```python
from build123d import *

# Parameters (mm, degrees)
RESSALTO_EXTRUS_O1_DEPTH = 8
ESBO_O2_W                = 2.8
ESBO_O2_H                = 2.8
CORTE_EXTRUS_O2_DEPTH    = 20.45530599


with BuildPart() as part:
    # Esboço1 → Ressalto-extrusão1 (new body)
    with BuildSketch(Plane.XY):
        with BuildLine():
            Line((0, 0), (-4.7, 0))
            Line((-4.7, 0), (-4.7, -2.5))
            Line((-4.7, -2.5), (-0.2, -2.5))
            Line((-0.2, -2.5), (14.8, -2.5))
            Line((14.8, -2.5), (14.8, 0))
            Line((14.8, 0), (13.3, 0))
            Line((13.3, 0), (13.3, 6))
            ThreePointArc((13.3, 6), (13, 7.270820393), (12.7, 6))
            Line((12.7, 6), (12.7, 0))
            Line((12.7, 0), (11.4, 0))
            Line((11.4, 0), (11.4, 6))
            ThreePointArc((11.4, 6), (11.1, 7.270820393), (10.8, 6))
            Line((10.8, 6), (10.8, 0))
            Line((10.8, 0), (9.5, 0))
            Line((9.5, 0), (9.5, 6))
            ThreePointArc((9.5, 6), (9.2, 7.270820393), (8.9, 6))
            Line((8.9, 6), (8.9, 0))
            Line((8.9, 0), (7.6, 0))
            Line((7.6, 0), (7.6, 6))
            ThreePointArc((7.6, 6), (7.3, 7.270820393), (7, 6))
            Line((7, 6), (7, 0))
            Line((7, 0), (5.7, 0))
            Line((5.7, 0), (5.7, 6))
            ThreePointArc((5.7, 6), (5.4, 7.270820393), (5.1, 6))
            Line((5.1, 6), (5.1, 0))
            Line((5.1, 0), (3.8, 0))
            Line((3.8, 0), (3.8, 6))
            ThreePointArc((3.8, 6), (3.5, 7.270820393), (3.2, 6))
            Line((3.2, 6), (3.2, 0))
            Line((3.2, 0), (1.9, 0))
            Line((1.9, 0), (1.3, 0))
            Line((1.3, 0), (0, 0))
        make_face()
    extrude(amount=RESSALTO_EXTRUS_O1_DEPTH)

    # Esboço2 → Corte-extrusão2 (cut, through all)
    with BuildSketch(Plane.XZ.offset(2.5)):
        with BuildLine():
            Line((-2.7, 8), (-4.7, 8))
            Line((-4.7, 8), (-4.7, 6))
            ThreePointArc((-4.7, 6), (-4.114213562, 7.414213562), (-2.7, 8))
        make_face()
        with BuildLine():
            Line((-4.7, 2), (-4.7, 0))
            Line((-4.7, 0), (-2.7, 0))
            ThreePointArc((-2.7, 0), (-4.114213562, 0.585786438), (-4.7, 2))
        make_face()
        with Locations((-0.7, 4)):
            Rectangle(ESBO_O2_W, ESBO_O2_H)
        with BuildLine():
            Line((13.8, 8), (14.8, 8))
            Line((14.8, 8), (14.8, 7))
            ThreePointArc((14.8, 7), (14.507106781, 7.707106781), (13.8, 8))
        make_face()
        with BuildLine():
            Line((13.8, 0), (14.8, 0))
            Line((14.8, 0), (14.8, 1))
            ThreePointArc((14.8, 1), (14.507106781, 0.292893219), (13.8, 0))
        make_face()
    extrude(amount=-CORTE_EXTRUS_O2_DEPTH, mode=Mode.SUBTRACT)


solid = part.part
```
For this review, take the finished solid that the model builds, in its own axes (mm). A direction names the side the tool comes from. Give positions to 0.01 mm unless a question says otherwise; leave off trailing zeros. Write each loop counter-clockwise with the first axis right and the second up, starting at its lowest first coordinate (ties: lowest second). Pieces come first, ordered by that corner, then holes.
Item 1: Wall thickness on probe 1 along X at (y, z) = (0.75, 1.75); probe 2 along X at (y, z) = (-1, 5.25); probe 3 along Z at (x, y) = (-2, -2): over which ranges is each line inside the solid? List them lowest first.
Item 2: Take a section at A-A (y = -0.25). Give the boundary of the cut face in (x, z).
Item 3: The part is to be moulded in two halves that separate along Y. For faces 5 (the face through (14.8, -1, 4)), 6 (the face through (5, -2.5, 4)), 7 (the face through (5.7, 3, 4)), say which applies: +Y half, -Y half, draft (parallel to the pull), parting line (faces both ways), or undercut.
Item 4: Machinability: for faces 1 (the face through (-1, -1, 2.6)), 2 (the face through (7.3, 2.5, 8)), 3 (the face through (3.2, 3, 4)), 4 (the face through (9.5, 3, 4)), which of the approach directions +Z, -Z, +X, -X, +Y, -Y give a long, thin tool a straight path to every point of the face, cutting with its end or side? Answer none if there is none.
Item 5: Take a section at C-C (x = 0.5). Give the boundary of the cut face in (y, z).
Item 6: Take a section at D-D (y = 6.6). Give the boundary of the cut face in (x, z), and give its area (3 significant figures).
Item 7: Insertion check: P1, Ø3, axis at y = 2, z = 5, coming from the +X side; P2, Ø0.6, axis at x = 6, z = 4, coming from the +Y side; P3, Ø1, axis at x = 10.5, z = 4, coming from the +Y side. Each pin has a flat end and moves straight along its axis. Give the tip position at first contact, or say it passes through.
Established:
1. probe 1: x = 3.2 to 3.8, 5.1 to 5.7, 7 to 7.6, 8.9 to 9.5, 10.8 to 11.4, 12.7 to 13.3
1. probe 2: x = -4.7 to -2.1, 0.7 to 14.8
1. probe 3: z = 0 to 2.6, 5.4 to 8
2. outline: (-4.7, 2) arc R2 ccw to (-2.7, 0) - (13.8, 0) arc R1 ccw to (14.8, 1) - (14.8, 7) arc R1 ccw to (13.8, 8) - (-2.7, 8) arc R2 ccw to (-4.7, 6) - close; hole (-2.1, 2.6) - (0.7, 2.6) - (0.7, 5.4) - (-2.1, 5.4) - close
3. face 5: draft
3. face 6: -Y half
3. face 7: undercut
4. face 1: +Y, -Y
4. face 2: +Z, +X, -X, +Y, -Y
4. face 3: +Z, -Z, -X
4. face 4: +Z, -Z
5. outline: (-2.5, 0) - (0, 0) - (0, 2.6) - (-2.5, 2.6) - close; (-2.5, 5.4) - (0, 5.4) - (0, 8) - (-2.5, 8) - close
6. outline: (2.83, 0) - (4.17, 0) - (4.17, 8) - (2.83, 8) - close; (4.73, 0) - (6.07, 0) - (6.07, 8) - (4.73, 8) - close; (6.63, 0) - (7.97, 0) - (7.97, 8) - (6.63, 8) - close; (8.53, 0) - (9.87, 0) - (9.87, 8) - (8.53, 8) - close; (10.43, 0) - (11.77, 0) - (11.77, 8) - (10.43, 8) - close; (12.33, 0) - (13.67, 0) - (13.67, 8) - (12.33, 8) - close
6. area: 64.4 mm2
7. P1: stops at x = 13.3
7. P2: stops at y = 7.2
7. P3: stops at y = 7.26
